The model under review builds one solid part; all positions refer to its coordinate system, in mm. A direction names the side the tool comes from. Coordinates: 2 decimals unless noted, no trailing zeros. Order: outer loops, then holes, each group sorted by start corner. A loop starts at its lowest first (then second) coordinate and runs counter-clockwise, first axis right, second up. Notation, with made-up numbers: (-16, 33) -> (-4, 33) arc R18 ccw to (-4, 60) -> close; hole circle Ø6 at (76, 45.5). An arc over 180 degrees is marked (long way). Use one line per item in the form item = value. Start each with the question number.
(1) Mouldability with a two-part tool opening along Y and no side actions: class faces 3 (the flat face through (1.1, -1.3, 0)), 4 (the cylindrical face through (0.748, -0.976, 2.634)), 5 (the flat face through (1.36, 2.39, 7.4)) as +Y half, -Y half, draft (parallel to the pull), parting line (faces both ways), or undercut.
(2) For faces 1 (the cylindrical face through (-1.5, -0.07, 17.32)), 2 (the cylindrical face through (-1.363, -2.319, 0.057)), list the 3-axis set-ups (+Z, -Z, +X, -X, +Y, -Y) from which the entire face can be reached by the end or side of a thin tool; tool diameter is ignored.
(3) Take a section at B-B (z = 18.75). State the section outline as (x, y) points, then the cut area to 3 significant figures.
(4) Take a section at A-A (z = 7.75). State the section outline as (x, y) points.
(5) Insertion check: pin 1 Ø1 at (x, z) = (2, 14.5) entering from +Y; pin 2 Ø1.5 at (y, z) = (2, 17) entering from +X. Each pin has a flat end and moves straight along its axis. Give the tip position at first contact, or say it passes through.
(6) Wall thickness on line 1 along X through (y, z) = (0, 2.2); line 2 along Z through (x, y) = (-1.75, 0.5); line 3 along Y through (x, z) = (0.8, 1.5): over which ranges is each line inside the solid? List them lowest first.
Autodesk Inventor part; units mm, degrees
ref_plane "YZ Plane" through (0, 0, 0) normal (1, 0, 0) x (0, 1, 0)
ref_plane "XZ Plane" through (0, 0, 0) normal (0, 1, 0) x (-1, 0, 0)
ref_plane "XY Plane" through (0, 0, 0) normal (0, 0, 1) x (1, 0, 0)
sketch "スケッチ1" plane through (0, 0, 0) normal (0, 0, 1) x (1, 0, 0)
  line L0 (0, 3.1754) -> (2.75, 1.5877)
  line L1 (2.75, 1.5877) -> (2.75, -1.5877)
  line L2 (2.75, -1.5877) -> (0, -3.1754)
  line L3 (0, -3.1754) -> (-2.75, -1.5877)
  line L4 (-2.75, -1.5877) -> (-2.75, 1.5877)
  line L5 (-2.75, 1.5877) -> (0, 3.1754)
  point P0 (0, 0)
  point P1 (0, 0)
  dimension "d0" = 5.5
extrude "押し出し1" add sketch "スケッチ1" along normal blind 15
sketch "スケッチ2" plane through (0, 0, 15) normal (0, 0, 1) x (1, 0, 0)
  circle A0 centre (0, 0) radius 1.5
  dimension "d3" = 3
extrude "押し出し2" add sketch "スケッチ2" along normal blind 5
thread "ねじ1"
chamfer "面取り1" distance 0.3 angle 45 1 edges at (-1.5, 0, 20)
fillet "フィレット1" radius 0.2 18 edges at (-1.375, 2.3816, 15) (1.375, 2.3816, 15) (2.75, 0, 15) (1.375, -2.3816, 15) (-1.375, -2.3816, 15) (-2.75, 0, 15) (-2.75, -1.5877, 7.5) (0, -3.1754, 7.5) (2.75, -1.5877, 7.5) (2.75, 1.5877, 7.5) (0, 3.1754, 7.5) (-2.75, 1.5877, 7.5) (-1.375, 2.3816, 0) (1.375, 2.3816, 0) (2.75, 0, 0) (1.375, -2.3816, 0) (-1.375, -2.3816, 0) (-2.75, 0, 0)
sketch "スケッチ3" plane through (0, 0, 0) normal (0, 0, -1) x (-1, 0, 0)
  point P0 (0, 0)
hole "穴1" at (0, 0, 0) direction (0, 0, 1) diameter 2.459 depth 5 tip angle 118
chamfer "面取り2" distance 0.2 angle 45 1 edges at (0, -1.2295, 0)
properties part number "hexagonal_spacer_M3_15mm" material "鋼、炭素鋼"
Findings:
q1.face_3 = draft
q1.face_4 = undercut
q1.face_5 = +Y half
q2.face_1 = +Z
q2.face_2 = -Z, -X, -Y
q3.outline = circle Ø3 at (0, 0)
q3.area = 7.07 mm²
q4.outline = (-2.75, -1.47) arc R0.2 ccw to (-2.65, -1.65) -> (-0.1, -3.12) arc R0.2 ccw to (0.1, -3.12) -> (2.65, -1.65) arc R0.2 ccw to (2.75, -1.47) -> (2.75, 1.47) arc R0.2 ccw to (2.65, 1.65) -> (0.1, 3.12) arc R0.2 ccw to (-0.1, 3.12) -> (-2.65, 1.65) arc R0.2 ccw to (-2.75, 1.47) -> close
q5.pin_1 = 2.31
q5.pin_2 = 0.83
q6.line_1 = -2.75 to -1.23, 1.23 to 2.75
q6.line_2 = 0 to 15
q6.line_3 = -2.71 to -0.93, 0.93 to 2.71
